Autodesk Inventor part; units mm, degrees
ref_plane "YZ Plane" through (0, 0, 0) normal (1, 0, 0) x (0, 1, 0)
ref_plane "XZ Plane" through (0, 0, 0) normal (0, 1, 0) x (-1, 0, 0)
ref_plane "XY Plane" through (0, 0, 0) normal (0, 0, 1) x (1, 0, 0)
sketch "Sketch1" plane through (0, 0, 0) normal (0, 0, 1) x (1, 0, 0)
  circle A0 centre (9.9098, 12.6224) radius 2.0828
  circle A1 centre (9.9098, -12.7776) radius 2.0828
  arc A2 (16.2598, 12.6224) -> (13.495, 17.8634) centre (9.9098, 12.6224) ccw
  arc A3 (3.5598, -12.7776) -> (16.2598, -12.7776) centre (9.9098, -12.7776) ccw
  line L0 (3.5598, 12.6224) -> (3.5598, -12.7776)
  line L1 (16.2598, 12.6224) -> (16.2598, -12.7776)
  circle A4 centre (-1.2027, 22.1474) radius 2.0828
  arc A5 (1.4862, 26.0782) -> (-1.2027, 17.3849) centre (-1.2027, 22.1474) ccw
  arc A6 (3.5598, 12.6224) -> (-1.2027, 17.3849) centre (-1.2027, 12.6224) ccw
  line L2 (1.4862, 26.0782) -> (13.495, 17.8634)
  point P0 (0, 0)
  dimension "d0" = 4.1656
  dimension "d1" = 12.7
  dimension "d2" = 9.525
extrude "Extrusion1" add sketch "Sketch1" along normal blind 1.5875
properties part number "brace_gusset" material "Acetal Resin, White"
Verification items for the finished model (mm, model axes). A direction names the side the tool comes from. Give positions to 0.01 mm unless a question says otherwise; leave off trailing zeros. Write each loop counter-clockwise with the first axis right and the second up, starting at its lowest first coordinate (ties: lowest second). Pieces come first, ordered by that corner, then holes.
(1) Cross-section at A-A (x = 11). Enter the section's corners in (y, z).
(2) Mould release check, pull along X, two halves, no side actions. Record for faces 1 (the face through (7.407, 22.028, 0.783)), 2 (the face through (11.03, 10.866, 0.783)), 3 (the face through (7, 4, 0)): +X half, -X half, draft (parallel to the pull), parting line (faces both ways), or undercut.
(3) Cross-section at C-C (z = 1.1). State how many separate pieces and enclosed holes the cut face has, plus the area to 3 significant figures.
(4) Gauge pin test, flat end, axial feed: pin 1 (0.5 mm diameter, centred on y = -1.5, z = 1, fed in from -X). Record the tip position at first contact, or that the pin passes through.
(5) Material ranges on line 1 (Y direction, x = 8.75, z = 1.1); line 2 (Y direction, x = 11, z = 1.2); line 3 (X direction, y = -12, z = 0.7), recorded low to high.
(6) Access from +Z, -Z, +X, -X, +Y, -Y to the whole of each face (thin tool, end or side, straight path). Record for faces 4 (the face through (3.56, 0, 1)), 5 (the face through (7, 4, 1.588)).
(7) Cross-section at B-B (y = -13.5). Enter the section's corners in (x, z), plus the area to 3 significant figures.
(8) Cross-section at D-D (x = 8.5). Enter the section's corners in (y, z).
Worked out:
1. outline: (-19.03, 0) - (-14.55, 0) - (-14.55, 1.59) - (-19.03, 1.59) - close; (-11, 0) - (10.85, 0) - (10.85, 1.59) - (-11, 1.59) - close; (14.4, 0) - (19.57, 0) - (19.57, 1.59) - (14.4, 1.59) - close
2. face 1: +X half
2. face 2: undercut
2. face 3: draft
3. separate pieces: 1
3. enclosed holes: 3
3. area: 523 mm2
4. pin 1: stops at x = 3.56
5. line 1: y = -19.02 to -14.51, -11.05 to 10.89, 14.35 to 21.11
5. line 2: y = -19.03 to -14.55, -11 to 10.85, 14.4 to 19.57
5. line 3: x = 3.56 to 7.98, 11.84 to 16.26
6. face 4: +Z, -Z, -X, -Y
6. face 5: +Z, +X, -X, +Y, -Y
7. outline: (3.6, 0) - (7.96, 0) - (7.96, 1.59) - (3.6, 1.59) - close; (11.86, 0) - (16.22, 0) - (16.22, 1.59) - (11.86, 1.59) - close
7. area: 13.8 mm2
8. outline: (-18.97, 0) - (-14.31, 0) - (-14.31, 1.59) - (-18.97, 1.59) - close; (-11.24, 0) - (11.09, 0) - (11.09, 1.59) - (-11.24, 1.59) - close; (14.16, 0) - (21.28, 0) - (21.28, 1.59) - (14.16, 1.59) - close
